Autodesk Inventor part; units mm, degrees
ref_plane "YZ Plane" through (0, 0, 0) normal (1, 0, 0) x (0, 1, 0)
ref_plane "XZ Plane" through (0, 0, 0) normal (0, 1, 0) x (-1, 0, 0)
ref_plane "XY Plane" through (0, 0, 0) normal (0, 0, 1) x (1, 0, 0)
sketch "Szkic1" plane through (0, 0, 0) normal (0, 0, 1) x (1, 0, 0)
  line L0 (0, -7.56) -> (0, 0)
  line L1 (0, 19.4) -> (0, 26.96)
  line L2 (-4.2, 4.2) -> (-11.76, 4.2)
  line L3 (-11.76, 15.2) -> (-4.2, 15.2)
  line L4 (15.2, 15.2) -> (22.76, 15.2)
  line L5 (15.2, 4.2) -> (22.76, 4.2)
  line L6 (-4.2, 26.96) -> (-4.2, 19.4)
  line L7 (-4.2, 19.4) -> (-11.76, 19.4)
  line L8 (-4.2, 15.2) -> (-4.2, 4.2)
  line L9 (-4.2, 0) -> (-4.2, -7.56)
  line L10 (-11.76, 0) -> (-4.2, 0)
  line L11 (15.2, -7.56) -> (11, -7.56)
  line L12 (0, -7.56) -> (-4.2, -7.56)
  line L13 (0, 0) -> (11, 0)
  line L14 (15.2, 0) -> (22.76, 0)
  line L15 (11, 26.96) -> (11, 19.4)
  line L16 (11, 0) -> (11, -7.56)
  line L17 (15.2, -7.56) -> (15.2, 0)
  line L18 (15.2, 4.2) -> (15.2, 15.2)
  line L19 (15.2, 19.4) -> (15.2, 26.96)
  line L20 (22.76, 19.4) -> (15.2, 19.4)
  line L21 (11, 19.4) -> (0, 19.4)
  line L22 (22.76, 19.4) -> (22.76, 15.2)
  line L23 (22.76, 4.2) -> (22.76, 0)
  line L24 (-4.2, 26.96) -> (0, 26.96)
  line L25 (11, 26.96) -> (15.2, 26.96)
  line L26 (-11.76, 0) -> (-11.76, 4.2)
  line L27 (-11.76, 15.2) -> (-11.76, 19.4)
  circle A0 centre (5.5, 9.7) radius 2.3
  dimension "d0" = 4.6
extrude "Wyciągnięcie proste1" add sketch "Szkic1" along normal blind 10
sketch "Szkic2" plane through (-11.76, 19.4, 0) normal (0, 1, 0) x (1, 0, 0)
  line L0 (7.56, 0) -> (0, 0)
  line L1 (0, 0) -> (0, -10)
  line L2 (7.56, -10) -> (0, -10)
  line L3 (7.56, 0) -> (7.56, -10)
  line L4 (34.52, 0) -> (26.96, 0)
  line L5 (26.96, 0) -> (26.96, -10)
  line L6 (34.52, -10) -> (26.96, -10)
  line L7 (34.52, 0) -> (34.52, -10)
  line L8 (0, 0) -> (0, -10)
  line L9 (0, -5) -> (3.4, -5)
  line L10 (34.52, 0) -> (34.52, -10)
  line L11 (34.52, -5) -> (31.12, -5)
  circle A0 centre (3.4, -5) radius 1.75
  circle A1 centre (31.12, -5) radius 1.75
  point P0 (11.76, 0)
  dimension "d3" = 3.4
  dimension "d4" = 3.4
  dimension "d5" = 3.5
  dimension "d6" = 3.5
extrude "Wyciągnięcie proste2" cut sketch "Szkic2" against normal through all contours A0 | A1
sketch "Szkic3" plane through (-4.2, -7.56, 0) normal (-1, 0, 0) x (0, 0, 1)
  line L0 (0, 7.56) -> (0, 0)
  line L1 (0, 0) -> (10, 0)
  line L2 (10, 7.56) -> (10, 0)
  line L3 (0, 7.56) -> (10, 7.56)
  line L4 (0, 34.52) -> (0, 26.96)
  line L5 (0, 26.96) -> (10, 26.96)
  line L6 (10, 34.52) -> (10, 26.96)
  line L7 (0, 34.52) -> (10, 34.52)
  line L8 (5, 0) -> (5, 3.4)
  line L9 (0, 34.52) -> (10, 34.52)
  line L10 (5, 34.52) -> (5, 31.12)
  circle A0 centre (5, 3.4) radius 1.75
  circle A1 centre (5, 31.12) radius 1.75
  point P0 (0, 7.56)
  dimension "d9" = 3.4
  dimension "d10" = 3.4
  dimension "d11" = 3.5
  dimension "d12" = 3.5
extrude "Wyciągnięcie proste3" cut sketch "Szkic3" against normal through all contours A0 | A1
chamfer "Faza2" distance 1 angle 45 4 edges at (-4.2, -4.16, 3.25) (17.61, 0, 5) (15.2, 23.56, 3.25) (-10.11, 19.4, 5)
sketch "Szkic8" plane through (15.2, -7.56, 0) normal (1, 0, 0) x (0, 0, -1)
  circle A0 centre (-5, 3.4) radius 1.75
  circle A1 centre (-5, 3.4) radius 1.5
  point P0 (0, 7.56)
  dimension "d42" = 3
extrude "Wyciągnięcie proste8" add sketch "Szkic8" against normal up to surface (4.2 mm away)
pattern_circular "Szyk kołowy3" count 4 over 360 about axis through (5.5, 9.7, 0) along (0, 0, 1) of "Wyciągnięcie proste8"
chamfer "Faza3" distance 0.2 angle 45 4 edges at (11, -4.16, 6.5) (-8.36, 4.2, 6.5) (0, 23.56, 6.5) (19.36, 15.2, 6.5)
properties part number "GripperMotorHinges"
Read the model definition and answer for the solid it produces. Units are mm, in the model's axes. A direction names the side the tool comes from. Give positions to 0.01 mm unless a question says otherwise; leave off trailing zeros. Write each loop counter-clockwise with the first axis right and the second up, starting at its lowest first coordinate (ties: lowest second). Pieces come first, ordered by that corner, then holes. Notation, with made-up numbers: (44.25, -31) -> (57.25, -31) arc R30 ccw to (57.25, 0) -> close; hole circle Ø5 at (85.5, -39.75). An arc over 180 degrees is marked (long way). Answer as a JSON object with one key per item and string values.
1) Flat-ended cylindrical pins translate along their axes: pin 1 Ø5 at (x, z) = (7.5, 2.5) entering from +Y; pin 2 Ø2 at (y, z) = (7.5, 8.5) entering from +X; pin 3 Ø2.5 at (y, z) = (-4.16, 5) entering from +X; pin 4 Ø4 at (y, z) = (23.56, 5) entering from -X. Find the tip coordinate at first contact, or state that the pin passes through.
Findings below:
{"pin 1": "stops at y = 19.4", "pin 2": "stops at x = 15.2", "pin 3": "passes through", "pin 4": "stops at x = -4.2"}
2) For a pull along X with two mould halves and no side action, classify faces 1 (the cylindrical face through (5.2, 7.42, 4.93)), 2 (the cylindrical face through (13.228, -5.624, 5.325)), 3 (the flat face through (-4.2, 22, 4)) as pulls with the +X half, pulls with the -X half, needs draft (parallel to the pull), parting line crosses it, or undercut.
Findings below:
{"face 1": "undercut", "face 2": "needs draft", "face 3": "pulls with the -X half"}
3) Section B-B on x = 19.36 is taken. Write down the section's boundary in (y, z).
Findings below:
{"outline": "(0, 0) -> (4.2, 0) -> (4.2, 3.25) -> (1, 3.25) -> (0, 2.25) -> close; (0, 7.75) -> (1, 6.75) -> (4.2, 6.75) -> (4.2, 10) -> (0, 10) -> close; (15.2, 0) -> (19.4, 0) -> (19.4, 3.5) -> (15.4, 3.5) -> (15.2, 3.3) -> close; (15.2, 6.7) -> (15.4, 6.5) -> (19.4, 6.5) -> (19.4, 10) -> (15.2, 10) -> close"}
4) A tool of negligible diameter and unlimited length cuts with its end or side. For faces 4 (the cylindrical face through (-1.62, -4.08, 3.25)), 5 (the flat face through (11, -2, 5)), 6 (the flat face through (6, 19.4, 5)), from which of +Z, -Z, +X, -X, +Y, -Y can it reach the whole face along a straight path? Write none if from no direction.
Findings below:
{"face 4": "-X", "face 5": "+Z, -Z, -Y", "face 6": "+Z, -Z, +Y"}
5) Section D-D on y = 23.56 is taken. Write down the section's boundary in (x, z), then the cut area to 3 significant figures.
Findings below:
{"outline": "(-4.2, 0) -> (0, 0) -> (0, 3.3) -> (-0.2, 3.5) -> (-4.2, 3.5) -> close; (-4.2, 6.5) -> (-0.2, 6.5) -> (0, 6.7) -> (0, 10) -> (-4.2, 10) -> close; (11, 0) -> (15.2, 0) -> (15.2, 2.25) -> (14.2, 3.25) -> (11, 3.25) -> close; (11, 6.75) -> (14.2, 6.75) -> (15.2, 7.75) -> (15.2, 10) -> (11, 10) -> close", "area": "55.7 mm^2"}
6) Section C-C on z = 5 is taken. Count the separate pieces of the cut face and the enclosed holes in it, then the cut area to 3 significant figures.
Findings below:
{"separate pieces": "9", "enclosed holes": "1", "area": "500 mm^2"}
7) Straight lines are drawn through the part: probe 1 along X at (y, z) = (17.5, 5); probe 2 along X at (y, z) = (1.95, 5); probe 3 along Y at (x, z) = (-0.9, 5). For each, find the intervals that lie inside material, in ascending order. Write a range as from..to.
Findings below:
{"probe 1": "x = -11.76..-10.11, -6.61..17.86, 20.86..22.76", "probe 2": "x = -11.76..-9.86, -6.86..17.61, 21.11..22.76", "probe 3": "y = -7.56..-5.91, -2.41..22.06, 25.06..26.96"}
8) Section A-A on y = -1 is taken. Write down the section's boundary in (x, z), then the cut area to 3 significant figures.
Findings below:
{"outline": "(-4.2, 0) -> (0, 0) -> (0, 10) -> (-4.2, 10) -> close; (11, 0) -> (15.2, 0) -> (15.2, 10) -> (11, 10) -> close", "area": "84.0 mm^2"}
